Work out the finished part from the listing and answer in its coordinate system (mm). Coordinates: 2 decimals unless noted, no trailing zeros. Write each loop counter-clockwise with the first axis right and the second up, starting at its lowest first coordinate (ties: lowest second). Pieces come first, ordered by that corner, then holes. Notation, with made-up numbers: (-32.75, 57) - (-25.75, 57) arc R23 ccw to (-25.75, 90) - close; hole circle Ø9 at (85, 58). An arc over 180 degrees is marked (long way). Use a Markdown table: item, result. Add a question column.
(1) The part is cut by section B-B, the plane y = 3.25. State how many separate pieces and enclosed holes the cut face has, then the cut area to 3 significant figures.
(2) The part is cut by section A-A, the plane z = -107.95. Give the vertices of the cut face in (x, y), then the cut area to 3 significant figures.
(3) The part is cut by section C-C, the plane x = 35. Give the vertices of the cut face in (y, z) (3 decimals).
(4) The part is cut by section D-D, the plane x = -36.5. Give the vertices of the cut face in (y, z) (3 decimals), then the cut area to 3 significant figures.
(5) Given pin 1 Ø3 at (x, z) = (-63.5, -12.7) entering from +Y; pin 2 Ø3 at (y, z) = (3, -98.5) entering from -X, each flat-ended and moving along its own axis, determine where each tip first touches the part or whether it passes through.
(6) Find the intervals of material crossed by line 1 (X direction, y = 2, z = -12.7); line 2 (Z direction, x = 45.5, y = 6.25) (3 decimals); line 3 (Z direction, x = -42, y = 4.75) (3 decimals), in increasing order. Write a range as from..to.
from build123d import *

# Parameters (mm, degrees)
BOSS_EXTRUDE1_DEPTH        = 6.35
SKETCH4_R                  = 14.2875
CUT_EXTRUDE2_DEPTH         = 135.10382172
SKETCH5_R                  = 4.7625
CUT_EXTRUDE3_DEPTH         = 50.8
F_10_CLEARANCE_HOLE1_D     = 5.1054
F_10_CLEARANCE_HOLE1_DEPTH = 50.8
F_10_CLEARANCE_HOLE1_TIP   = 1.533816902
FILLET1_R                  = 6.35
F_5_16_CLEARANCE_HOLE1_D   = 8.4328


with BuildPart() as part:
    # Sketch1 → Boss-Extrude1 (new body)
    with BuildSketch(Plane(origin=(0, 0, 0), x_dir=(1, 0, 0), z_dir=(0, 1, 0))):
        Polygon((-69.85, -19.05), (69.85, -19.05), (69.85, 57.15), (6.35, 114.3), (-6.35, 114.3), (-69.85, 57.15), align=None)
    extrude(amount=BOSS_EXTRUDE1_DEPTH)

    # Sketch4 → Cut-Extrude2 (cut, through all)
    with BuildSketch(Plane(origin=(0, 6.35, 0), x_dir=(1, 0, 0), z_dir=(0, 1, 0))):
        with Locations(Location((0, 63.5, 0), (0, 0, 270))):
            Circle(SKETCH4_R)
    extrude(amount=-CUT_EXTRUDE2_DEPTH, mode=Mode.SUBTRACT)

    # Sketch5 → Cut-Extrude3 (cut)
    with BuildSketch(Plane(origin=(0, 6.35, 19.05), x_dir=(-0.9584281674521108, 0, 0.2853339233851958), z_dir=(0, 1, 0))):
        with Locations(Location((21.697168114, -77.740965053, 0), (0, 0, 73.42119018))):
            Circle(SKETCH5_R)
        with Locations(Location((18.665649821, -27.031499499, 0), (0, 0, 73.42119018))):
            Circle(SKETCH5_R)
        with Locations(Location((-30.411025551, -12.420868461, 0), (0, 0, 73.42119018))):
            Circle(SKETCH5_R)
        with Locations(Location((-60.684163962, -53.21519516, 0), (0, 0, 73.42119018))):
            Circle(SKETCH5_R)
    extrude(amount=-CUT_EXTRUDE3_DEPTH, mode=Mode.SUBTRACT)

    # #10 Clearance Hole1
    with Locations(Plane(origin=(0, 6.35, 19.05), x_dir=(1, 0, 0), z_dir=(0, 1, 0))):
        with Locations((-63.5, 31.75), (63.5, 31.75), (0, 127)):
            Hole(F_10_CLEARANCE_HOLE1_D / 2, depth=F_10_CLEARANCE_HOLE1_DEPTH)
            with Locations((0, 0, -(F_10_CLEARANCE_HOLE1_DEPTH + F_10_CLEARANCE_HOLE1_TIP / 2))):  # 118° drill point
                Cone(0, F_10_CLEARANCE_HOLE1_D / 2, F_10_CLEARANCE_HOLE1_TIP, mode=Mode.SUBTRACT)

    # Fillet1
    fillet1_edges = [part.edges().sort_by_distance(p)[0] for p in [
        (-69.85, 3.175, -57.15),
        (-6.35, 3.175, -114.3),
        (6.35, 3.175, -114.3),
        (69.85, 3.175, -57.15),
        (69.85, 3.175, 19.05),
        (-69.85, 3.175, 19.05),
    ]]
    fillet(fillet1_edges, radius=FILLET1_R)

    # 5/16 Clearance Hole1 (through all)
    with Locations(Plane(origin=(0, 0, 19.05), x_dir=(-1, 0, 0), z_dir=(0, -1, 0))):
        with Locations((-44.45, 85.725), (44.45, 85.725), (0, 6.35)):
            Hole(F_5_16_CLEARANCE_HOLE1_D / 2)


solid = part.part
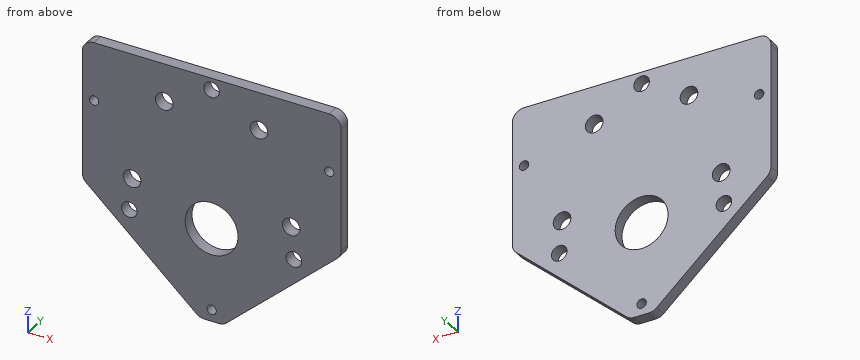
Model answer:
| question | item | result |
|---|---|---|
| 1 | separate pieces | 1 |
| 1 | enclosed holes | 11 |
| 1 | area | 13,800 mm^2 |
| 2 | outline | (-13.41, 0) - (-2.55, 0) - (-2.55, 6.35) - (-13.41, 6.35) - close; (2.55, 0) - (13.41, 0) - (13.41, 6.35) - (2.55, 6.35) - close |
| 2 | area | 138 mm^2 |
| 3 | outline | (0, -88.515) - (6.35, -88.515) - (6.35, 19.05) - (0, 19.05) - close |
| 4 | outline | (0, -87.165) - (6.35, -87.165) - (6.35, 19.05) - (0, 19.05) - close |
| 4 | area | 674 mm^2 |
| 5 | pin 1 | through |
| 5 | pin 2 | x = -25.57 |
| 6 | line 1 | -69.85..-66.05, -60.95..60.95, 66.05..69.85 |
| 6 | line 2 | -79.065..-70.759, -62.591..-53.308, -45.229..19.05 |
| 6 | line 3 | -82.215..-70.107, -63.243..-53.929, -44.607..19.05 |
